Here's how the part is built. I have some questions about the finished solid (model axes, mm). Face numbers are marked on the shaded views. A direction names the side the tool comes from. Give positions to 0.01 mm unless a question says otherwise; leave off trailing zeros. Write each loop counter-clockwise with the first axis right and the second up, starting at its lowest first coordinate (ties: lowest second). Pieces come first, ordered by that corner, then holes. Notation, with made-up numbers: M 77,53.5 L 123,53.5 A28 ccw 123,91.5 Z; hole C 49,76.5 d11. An arc over 180 degrees is marked long. Use one line per item in the form item = value. Start each with the question number.
from build123d import *

# Parameters (mm, degrees)
BOSS_EXTRUDE1_DEPTH = 23.5
SKETCH2_W           = 36
SKETCH2_H           = 39.6
BOSS_EXTRUDE2_DEPTH = 3
CUT_EXTRUDE3_REACH  = 67.916
SKETCH5_W           = 25
SKETCH5_H           = 19.5


with BuildPart() as part:
    # Sketch1 → Boss-Extrude1 (new body)
    with BuildSketch(Plane(origin=(0, 0, 0), x_dir=(1, 0, 0), z_dir=(0, 1, 0))):
        Polygon((-48.611740356, -17.456705616), (-48.611740356, -16.615368715), (-48.611740356, -14.456705616), (-48.611740356, -12.856705616), (-48.611740356, 16.143294384), (-48.611740356, 19.143294384), (-51.611740356, 19.143294384), (-51.611740356, -20.456705616), (-46.111740356, -20.456705616), (-46.111740356, -17.456705616), align=None)
        Polygon((-48.611740356, -12.856705616), (-48.611740356, -14.456705616), (-18.611740356, -14.456705616), (-18.611740356, -17.456705616), (-21.111740356, -17.456705616), (-21.111740356, -20.456705616), (-15.611740356, -20.456705616), (-15.611740356, 19.143294384), (-48.611740356, 19.143294384), (-48.611740356, 16.143294384), (-18.611740356, 16.143294384), (-18.611740356, -12.856705616), align=None)
    extrude(amount=BOSS_EXTRUDE1_DEPTH)

    # Sketch2 → Boss-Extrude2 (add)
    with BuildSketch(Plane.XZ):
        with Locations((-33.611740356, 0.656705616)):
            Rectangle(SKETCH2_W, SKETCH2_H)
    extrude(amount=BOSS_EXTRUDE2_DEPTH)

    # Sketch5 → Cut-Extrude3 (cut, up to next)
    with BuildSketch(Plane.XY.offset(14.456705616), mode=Mode.PRIVATE) as cut_extrude3_sk1:
        with Locations((-33.611740356, 13.75)):
            Rectangle(SKETCH5_W, SKETCH5_H)
    cut_extrude3_tool1 = extrude(cut_extrude3_sk1.sketch, amount=-CUT_EXTRUDE3_REACH, mode=Mode.PRIVATE) & part.part
    add(cut_extrude3_tool1.solids().sort_by_distance((-33.61174, 13.75, 14.456706))[0], mode=Mode.SUBTRACT)


solid = part.part
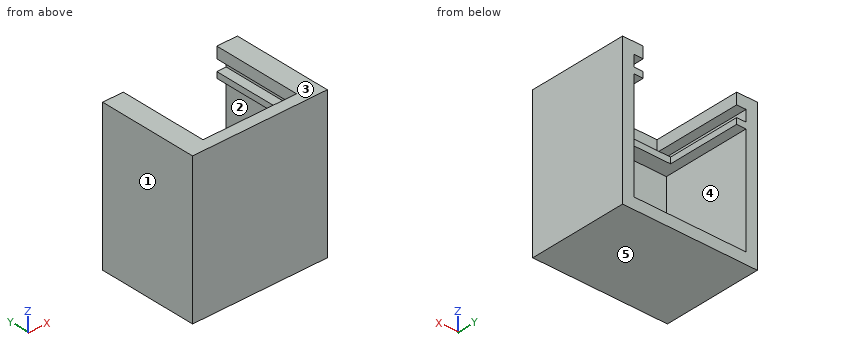
1) Suppose I cut it at B-B, the plane x = -20. List the corners of the cut face in (y, z) for me, and give its area (3 significant figures).
2) Thinking about a two-plate mould opening in X: for the marked faces 1, 2 and 3, which applies, released by +X, released by -X, zero draft, split by the parting line, or undercut?
3) On a 3-axis mill with a long thin cutter (end or side, diameter ignored), from which of +Z, -Z, +X, -X, +Y, -Y can I reach the whole of each face in a straight line? I mean the marked faces 4 and 5. Say none if no direction works.
4) Suppose I cut it at C-C, the plane y = 12. List the corners of the cut face in (x, z) for me.
5) Suppose I cut it at A-A, the plane z = -12.5. List the corners of the cut face in (x, y) for me, and give its area (3 significant figures).
6) Will these pins go through, and if not, where does the flat tip stop? P1, Ø3, axis at x = -33, z = 5, coming from the +Y side; P2, Ø1, axis at x = -28.5, y = 3.5, coming from the +Z side; P3, Ø7, axis at x = -36, y = 11, coming from the +Z side.
7) Suppose I cut it at D-D, the plane x = -42. List the corners of the cut face in (y, z) for me.
8) Please list where these lines run through material, in increasing order: line 1 (X direction, y = 17.5, z = -14.5); line 2 (X direction, y = 19, z = 13); line 3 (Z direction, x = -19, y = 2.25).
Checks:
q1.outline = M -3,-19.14 L 23.5,-19.14 L 23.5,-16.14 L 0,-16.14 L 0,12.86 L 23.5,12.86 L 23.5,14.46 L 0,14.46 L 0,17.46 L 23.5,17.46 L 23.5,20.46 L -3,20.46 Z
q1.area = 297 mm^2
q2.face_1 = released by -X
q2.face_2 = undercut
q2.face_3 = zero draft
q3.face_4 = +Y
q3.face_5 = -Z, +X, -X, +Y, -Y
q4.outline = M -51.61,-19.14 L -15.61,-19.14 L -15.61,20.46 L -21.11,20.46 L -21.11,17.46 L -18.61,17.46 L -18.61,14.46 L -21.11,14.46 L -21.11,12.86 L -18.61,12.86 L -18.61,-16.14 L -48.61,-16.14 L -48.61,12.86 L -46.11,12.86 L -46.11,14.46 L -48.61,14.46 L -48.61,17.46 L -46.11,17.46 L -46.11,20.46 L -51.61,20.46 Z
q5.outline = M -51.61,-3 L -15.61,-3 L -15.61,23.5 L -18.61,23.5 L -18.61,0 L -48.61,0 L -48.61,23.5 L -51.61,23.5 Z
q5.area = 249 mm^2
q6.P1 = 0
q6.P2 = 14.46
q6.P3 = -16.14
q7.outline = M -3,-19.14 L 23.5,-19.14 L 23.5,-16.14 L 0,-16.14 L 0,12.86 L 4,12.86 L 4,14.46 L 0,14.46 L 0,20.46 L -3,20.46 Z
q8.line_1 = -51.61 to -48.61, -18.61 to -15.61
q8.line_2 = -51.61 to -46.11, -21.11 to -15.61
q8.line_3 = -19.14 to -16.14, 12.86 to 14.46, 17.46 to 20.46
